```python
from build123d import *

# Parameters (mm, degrees)
SKETCH_1_R          = 25.5
SKETCH_1_R_2        = 23.5
EXTRUDE_1_DEPTH     = 10
EXTRUDE_2_DEPTH     = 10
SKETCH_3_R          = 2.25
CUT_EXTRUDE_1_DEPTH = 52
SKETCH_4_R          = 2.25
CUT_EXTRUDE_2_DEPTH = 52
SKETCH_7_W          = 24
SKETCH_7_H          = 3.731601122
SKETCH_7_W_2        = 3.731601122
SKETCH_7_H_2        = 24
CUT_EXTRUDE_4_DEPTH = 11.0000001


with BuildPart() as part:
    # 草图1 → 凸台-拉伸1 (new body)
    with BuildSketch(Plane(origin=(0, 0, 0), x_dir=(1, 0, 0), z_dir=(0, 1, 0))):
        Circle(SKETCH_1_R)
        Circle(SKETCH_1_R_2, mode=Mode.SUBTRACT)
    extrude(amount=EXTRUDE_1_DEPTH)

    # 草图2 → 凸台-拉伸2 (add)
    with BuildSketch(Plane(origin=(0, 10, 0), x_dir=(1, 0, 0), z_dir=(0, 1, 0))):
        with BuildLine():
            Line((-14, 25.5), (14, 25.5))
            Line((14, 25.5), (14, 20.205197351))
            ThreePointArc((14, 20.205197351), (0, 24.581497107), (-14, 20.205197351))
            Line((-14, 20.205197351), (-14, 25.5))
        make_face()
        with BuildLine():
            Line((20.205197351, 14), (25.5, 14))
            Line((25.5, 14), (25.5, -14))
            Line((25.5, -14), (20.205197351, -14))
            ThreePointArc((20.205197351, -14), (24.581497107, 0), (20.205197351, 14))
        make_face()
        with BuildLine():
            Line((14, -20.205197351), (14, -25.5))
            Line((14, -25.5), (-14, -25.5))
            Line((-14, -25.5), (-14, -20.205197351))
            ThreePointArc((-14, -20.205197351), (0, -24.581497107), (14, -20.205197351))
        make_face()
        with BuildLine():
            Line((-20.205197351, -14), (-25.5, -14))
            Line((-25.5, -14), (-25.5, 14))
            Line((-25.5, 14), (-20.205197351, 14))
            ThreePointArc((-20.205197351, 14), (-24.581497107, 0), (-20.205197351, -14))
        make_face()
    extrude(amount=-EXTRUDE_2_DEPTH)

    # 草图3 → 切除-拉伸1 (cut, through all)
    with BuildSketch(Plane.XY.offset(25.5)):
        with Locations((-6.75, 5)):
            Circle(SKETCH_3_R)
        with Locations((6.75, 5)):
            Circle(SKETCH_3_R)
    extrude(amount=-CUT_EXTRUDE_1_DEPTH, mode=Mode.SUBTRACT)

    # 草图4 → 切除-拉伸2 (cut, through all)
    with BuildSketch(Plane.ZY.offset(25.5)):
        with Locations((-6.75, 5)):
            Circle(SKETCH_4_R)
        with Locations((6.75, 5)):
            Circle(SKETCH_4_R)
    extrude(amount=-CUT_EXTRUDE_2_DEPTH, mode=Mode.SUBTRACT)

    # 草图7 → 切除-拉伸4 (cut, through all)
    with BuildSketch(Plane(origin=(0, 10, 0), x_dir=(1, 0, 0), z_dir=(0, 1, 0))):
        with Locations((0, 21.634199439)):
            Rectangle(SKETCH_7_W, SKETCH_7_H)
        with Locations((21.634199439, 0)):
            Rectangle(SKETCH_7_W_2, SKETCH_7_H_2)
        with Locations((0, -21.634199439)):
            Rectangle(SKETCH_7_W, SKETCH_7_H)
        with Locations((-21.634199439, 0)):
            Rectangle(SKETCH_7_W_2, SKETCH_7_H_2)
    extrude(amount=-CUT_EXTRUDE_4_DEPTH, mode=Mode.SUBTRACT)


solid = part.part
```
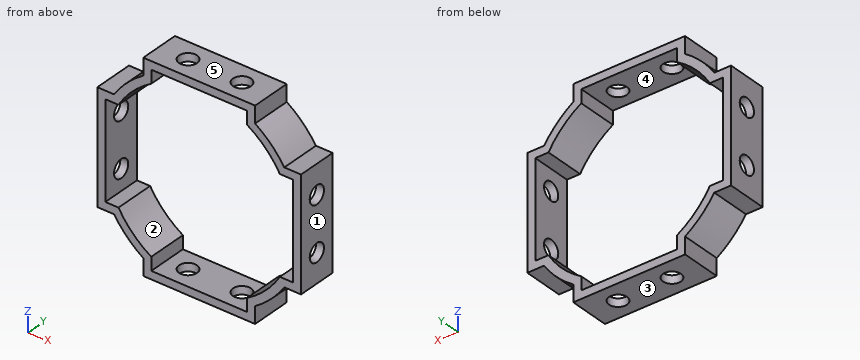
The model under review builds one solid part; all positions refer to its coordinate system, in mm. Face numbers are marked on the shaded views. A direction names the side the tool comes from. Round coordinates to 2 decimals unless told otherwise and drop trailing zeros. Loops run counter-clockwise (first coordinate to the right, second up) from the corner with the lowest first, then second, coordinate; pieces in that order, holes last.
Item 1: For line 1 (X direction, y = 8.5, z = -22); line 2 (Z direction, x = -7, y = 7.5), list the stretches that pass through material, from the lowest coordinate up.
Determined:
line 1: x = -14 to -12, 12 to 14
line 2: z = -25.5 to -23.5, 23.5 to 25.5
Item 2: Take a section at A-A (z = 0). Write out the cut boundary in (x, y), then the cut area to 3 significant figures.
Determined:
outline: (-25.5, 0) - (-23.5, 0) - (-23.5, 10) - (-25.5, 10) - close; (23.5, 0) - (25.5, 0) - (25.5, 10) - (23.5, 10) - close
area: 40.0 mm2
Item 3: Mouldability with a two-part tool opening along Z and no side actions: class the marked faces 1, 2 and 3 as released by +Z, released by -Z, zero draft, split by the parting line, or undercut.
Determined:
face 1: zero draft
face 2: undercut
face 3: released by -Z
Item 4: Take a section at D-D (x = 1). Write out the cut boundary in (y, z).
Determined:
outline: (0, -25.5) - (10, -25.5) - (10, -23.5) - (0, -23.5) - close; (0, 23.5) - (10, 23.5) - (10, 25.5) - (0, 25.5) - close
Item 5: Clearance check with flat-ended pins moving along their axes: pin 1 Ø3.5 at (x, y) = (22.5, 6.5) entering from -Z; pin 2 Ø1.5 at (x, y) = (19.5, 4) entering from +Z; pin 3 Ø12 at (x, z) = (-13.5, 14) entering from +Y; pin 4 Ø3.5 at (x, y) = (-22, 5.5) entering from +Z. State where each tip first meets the part, or that it passes through.
Determined:
pin 1: stops at z = -14.82
pin 2: stops at z = 17.28
pin 3: stops at y = 10
pin 4: stops at z = 15.5
Item 6: For the marked faces 4 and 5, list the 3-axis set-ups (+Z, -Z, +X, -X, +Y, -Y) from which the entire face can be reached by the end or side of a thin tool; tool diameter is ignored.
Determined:
face 4: +Y, -Y
face 5: +Z, +X, -X, +Y, -Y
Item 7: Take a section at B-B (x = -6.75). Write out the cut boundary in (y, z), then the cut area to 3 significant figures.
Determined:
outline: (0, -25.5) - (2.75, -25.5) - (2.75, -23.5) - (0, -23.5) - close; (0, 23.5) - (2.75, 23.5) - (2.75, 25.5) - (0, 25.5) - close; (7.25, -25.5) - (10, -25.5) - (10, -23.5) - (7.25, -23.5) - close; (7.25, 23.5) - (10, 23.5) - (10, 25.5) - (7.25, 25.5) - close
area: 22.0 mm2
